The model under review builds one solid part; all positions refer to its coordinate system, in mm. A direction names the side the tool comes from. Give positions to 0.01 mm unless a question says otherwise; leave off trailing zeros. Write each loop counter-clockwise with the first axis right and the second up, starting at its lowest first coordinate (ties: lowest second). Pieces come first, ordered by that corner, then holes. Notation, with made-up numbers: M 67.25,-30.75 L 114.25,-30.75 A20 cw 114.25,0.25 Z; hole C 25.25,86.25 d4. An arc over 180 degrees is marked long. Write each question's results on one line, items separated by ' | '. Start each with the question number.
from build123d import *

# Parameters (mm, degrees)
SKETCH1_R           = 7.5
BOSS_EXTRUDE1_DEPTH = 27
SKETCH2_R           = 5
CUT_EXTRUDE1_DEPTH  = 11
SKETCH3_R           = 1
CUT_EXTRUDE2_DEPTH  = 11
SKETCH4_R           = 1.6
CUT_EXTRUDE3_DEPTH  = 11
CHAMFER1_SIZE       = 1
CHAMFER1_SIZE2      = 1.732050808


with BuildPart() as part:
    # Sketch1 → Boss-Extrude1 (new body)
    with BuildSketch(Plane(origin=(0, 0, 0), x_dir=(1, 0, 0), z_dir=(0, 1, 0))):
        Circle(SKETCH1_R)
    extrude(amount=BOSS_EXTRUDE1_DEPTH)

    # Sketch2 → Cut-Extrude1 (cut)
    with BuildSketch(Plane.XZ):
        Circle(SKETCH2_R)
    extrude(amount=-CUT_EXTRUDE1_DEPTH, mode=Mode.SUBTRACT)

    # Sketch3 → Cut-Extrude2 (cut)
    with BuildSketch(Plane(origin=(0, 27, 0), x_dir=(1, 0, 0), z_dir=(0, 1, 0))):
        Circle(SKETCH3_R)
    extrude(amount=-CUT_EXTRUDE2_DEPTH, mode=Mode.SUBTRACT)

    # Sketch4 → Cut-Extrude3 (cut)
    with BuildSketch(Plane.XY):
        with Locations((0, 22)):
            Circle(SKETCH4_R)
        with Locations((0, 5)):
            Circle(SKETCH4_R)
    extrude(amount=-CUT_EXTRUDE3_DEPTH, mode=Mode.SUBTRACT)

    # Chamfer1
    chamfer1_edges = [part.edges().sort_by_distance(p)[0] for p in [
        (-5, 0, 0),
    ]]
    chamfer1_side = [part.faces().sort_by_distance(p)[0] for p in [
        (-7.287867966, 0, 0),
    ]]
    chamfer(chamfer1_edges, length=CHAMFER1_SIZE, length2=CHAMFER1_SIZE2, reference=chamfer1_side[0])


solid = part.part
(1) Add section D-D (y = 22). State the section outline as (x, z) points.
(2) Wall thickness on L1, parallel to Y at x = 0, z = -6.75; L2, parallel to Y at x = 0, z = -3.5; L3, parallel to Z at x = 0, y = 8: over which ranges is each line inside the solid? List them lowest first.
(3) Clearance check with flat-ended pins moving along their axes: P1, Ø9, axis at x = 0, z = 0, coming from the -Y side; P2, Ø1.6, axis at x = 0, z = 0, coming from the +Y side; P3, Ø3, axis at y = 8.5, z = -4.5, coming from the -X side. State where each tip first meets the part, or that it passes through.
(4) Machinability: for faces 4 (the cylindrical face through (1.48, 4.39, -6.1)), 5 (the flat face through (0, 16, 0)), 6 (the flat face through (0, 11, 0)), which of the approach directions +Z, -Z, +X, -X, +Y, -Y give a long, thin tool a straight path to every point of the face, cutting with its end or side? Answer none if there is none.
(5) Add section C-C (y = 11.5). State the section outline as (x, z) points, then the cut area to 3 significant figures.
(6) Add section B-B (y = 8.75). State the section outline as (x, z) points, then the cut area to 3 significant figures.
(7) Add section A-A (x = 0). State the section outline as (y, z) points.
(8) Draft analysis for pull direction X (two halves, no side actions). For faces 1 (the flat face through (2, 0, -6)), 2 (the cylindrical face through (-1.63, 13.31, 7.32)), 3 (the cylindrical face through (3, 6, 4)), state which applies: pulls with the +X half, pulls with the -X half, needs draft (parallel to the pull), parting line crosses it, or undercut.
Calculated:
1) outline: M -1.6,-7.33 L -1.6,0 L -1,0 A1 cw 1,0 L 1.6,0 L 1.6,-7.33 A7.5 ccw long Z
2) L1: y = 0 to 3.4, 6.6 to 20.4, 23.6 to 27 | L2: y = 11 to 20.4, 23.6 to 27 | L3: z = -7.5 to -5, 5 to 7.5
3) P1: stops at y = 11 | P2: stops at y = 16 | P3: stops at x = -6.87
4) face 4: -Z | face 5: +Y | face 6: -Y
5) outline: C 0,0 d15 | area: 177 mm²
6) outline: C 0,0 d15; hole C 0,0 d10 | area: 98.2 mm²
7) outline: M 0,-7.5 L 3.4,-7.5 L 3.4,-5 L 1.73,-5 L 0,-6 Z; M 0,6 L 1.73,5 L 11,5 L 11,-5 L 6.6,-5 L 6.6,-7.5 L 20.4,-7.5 L 20.4,-1 L 16,-1 L 16,1 L 27,1 L 27,7.5 L 0,7.5 Z; M 23.6,-7.5 L 27,-7.5 L 27,-1 L 23.6,-1 Z
8) face 1: needs draft | face 2: parting line crosses it | face 3: undercut
